Can you work these out from the drawing? Everything is in mm from the part's minimum corner. A direction names the side the tool comes from. Give positions to 0.01 mm unless a question says otherwise; leave off trailing zeros. Order: outer loops, then holes, each group sorted by start corner. A loop starts at its lowest first (then second) coordinate and runs counter-clockwise, first axis right, second up. Notation, with made-up numbers: M -40,-32 L -13,-32 A34 ccw -13,6 Z; hole C -35,69 d10. An arc over 180 degrees is marked long. Answer as a JSON object with one key per item and string values.
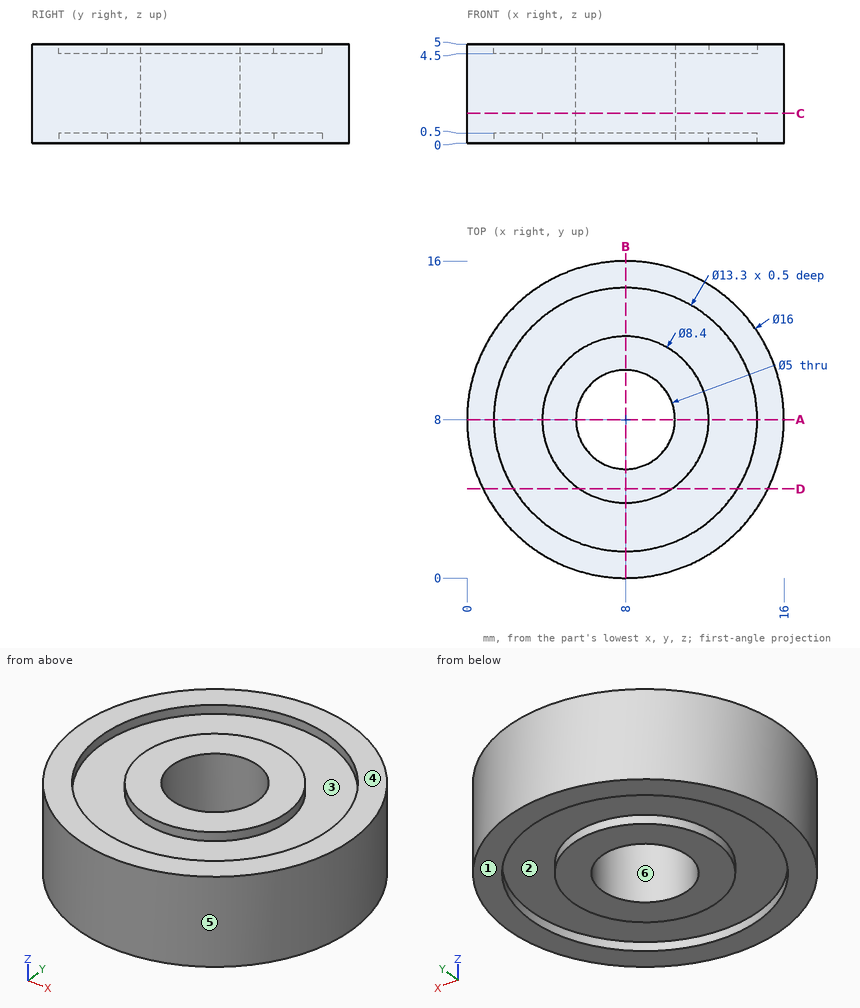
1) I need wall thicknesses on L1, parallel to Y at x = 9, z = 0.2; L2, parallel to Y at x = 8, z = 1.35; L3, parallel to X at y = 11, z = 4.7. Which ranges of each line are inside material? Lowest first, please.
Results found:
{"L1": "y = 0.06 to 1.43, 3.92 to 5.71, 10.29 to 12.08, 14.57 to 15.94", "L2": "y = 0 to 5.5, 10.5 to 16", "L3": "x = 0.58 to 2.07, 5.06 to 10.94, 13.93 to 15.42"}
2) I want a section at C-C on z = 1.5. Write out the boundary of the cut face in (x, y), and give its area (3 significant figures).
Results found:
{"outline": "C 8,8 d16; hole C 8,8 d5", "area": "181 mm²"}
3) Thinking about a two-plate mould opening in Y: for the marked faces 4, 5 and 6, which applies, pulls with the +Y half, pulls with the -Y half, needs draft (parallel to the pull), parting line crosses it, or undercut?
Results found:
{"face 4": "needs draft", "face 5": "parting line crosses it", "face 6": "undercut"}
4) For the marked faces 1, 2 and 3, which set-ups out of +Z, -Z, +X, -X, +Y, -Y let a thin tool reach every point of the face, with its end or its side?
Results found:
{"face 1": "-Z, +X, -X, +Y, -Y", "face 2": "-Z", "face 3": "+Z"}
5) I want a section at D-D on y = 4.5. Write out the boundary of the cut face in (x, z), and give its area (3 significant figures).
Results found:
{"outline": "M 0.81,0 L 2.35,0 L 2.35,0.5 L 5.68,0.5 L 5.68,0 L 10.32,0 L 10.32,0.5 L 13.65,0.5 L 13.65,0 L 15.19,0 L 15.19,5 L 13.65,5 L 13.65,4.5 L 10.32,4.5 L 10.32,5 L 5.68,5 L 5.68,4.5 L 2.35,4.5 L 2.35,5 L 0.81,5 Z", "area": "65.3 mm²"}
6) I'm going to push flat-ended pins straight in: pin 1 Ø3 at (x, z) = (12, 1.5) entering from -Y; pin 2 Ø1.5 at (y, z) = (14, 4) entering from +X; pin 3 Ø3 at (y, z) = (12, 3) entering from -X. Where does each tip first touch, or does it pass through?
Results found:
{"pin 1": "stops at y = 0.4", "pin 2": "stops at x = 14.04", "pin 3": "stops at x = 0.4"}
7) I want a section at A-A on y = 8. Write out the boundary of the cut face in (x, z).
Results found:
{"outline": "M 0,0 L 1.35,0 L 1.35,0.5 L 3.8,0.5 L 3.8,0 L 5.5,0 L 5.5,5 L 3.8,5 L 3.8,4.5 L 1.35,4.5 L 1.35,5 L 0,5 Z; M 10.5,0 L 12.2,0 L 12.2,0.5 L 14.65,0.5 L 14.65,0 L 16,0 L 16,5 L 14.65,5 L 14.65,4.5 L 12.2,4.5 L 12.2,5 L 10.5,5 Z"}
